Design review of the part built by this model. Coordinates are the model's own, in mm. Face numbers are marked on the shaded views. A direction names the side the tool comes from. Coordinates: 2 decimals unless noted, no trailing zeros. Write each loop counter-clockwise with the first axis right and the second up, starting at its lowest first coordinate (ties: lowest second). Pieces come first, ordered by that corner, then holes. Notation, with made-up numbers: M 69.5,66.25 L 116.5,66.25 A10 cw 116.5,79.25 Z; hole C 30,53 d6. An arc over 180 degrees is marked long. Return JSON: item names as keys, results as strings. Group by question number.
```python
from build123d import *

# Parameters (mm, degrees)
F1_DEPTH = 2
F3_DEPTH = 13
F4_W     = 5
F4_H     = 16
F5_DEPTH = 25
F6_R     = 4


with BuildPart() as f1:
    # F0 (on Top) → F1 (new body)
    with BuildSketch(Plane.XY):
        with BuildLine():
            ThreePointArc((0, -12), (-12, 5e-09), (9.9e-09, 12))
            Line((9.9e-09, 12), (-17, 12))
            Line((-17, 12), (-17, -12))
            Line((-17, -12), (0, -12))
        make_face()
        with BuildLine():
            ThreePointArc((0, -12), (8.4852813742, -8.4852813742), (12, 0))
            ThreePointArc((12, 0), (8.4852813777, 8.4852813707), (9.9e-09, 12))
            ThreePointArc((9.9e-09, 12), (-12, 5e-09), (0, -12))
        make_face()
    extrude(amount=F1_DEPTH)

    # F2 (on face) → F3 (join)
    with BuildSketch(Plane.XY.offset(2)):
        with BuildLine():
            Line((-13, 8), (0, 8))
            Line((0, 8), (8.94427191, 8))
            ThreePointArc((8.94427191, 8), (4.8989794901, 10.9544511481), (9.9e-09, 12))
            Line((9.9e-09, 12), (-17, 12))
            Line((-17, 12), (-17, -12))
            Line((-17, -12), (0, -12))
            ThreePointArc((0, -12), (4.8989794856, -10.9544511501), (8.94427191, -8))
            Line((8.94427191, -8), (0, -8))
            Line((0, -8), (-13, -8))
            Line((-13, -8), (-13, 8))
        make_face()
        with BuildLine():
            ThreePointArc((0, 8), (5.6568542495, 5.6568542495), (8, 0))
            ThreePointArc((8, 0), (5.6568542495, -5.6568542495), (0, -8))
            Line((0, -8), (8.94427191, -8))
            ThreePointArc((8.94427191, -8), (12, 0), (8.94427191, 8))
            Line((8.94427191, 8), (0, 8))
        make_face()
    extrude(amount=F3_DEPTH)

    # F4 (on face) → F5 (cut)
    with BuildSketch(Plane.XY.offset(2)):
        with Locations((-10.5, 0)):
            Rectangle(F4_W, F4_H)
    extrude(amount=-F5_DEPTH, mode=Mode.SUBTRACT)

    # F6
    f6_edges = [f1.edges().sort_by_distance(p)[0] for p in [
        (-17, 12, 7.5),
        (-17, -12, 7.5),
    ]]
    fillet(f6_edges, radius=F6_R)


solid = f1.part
```
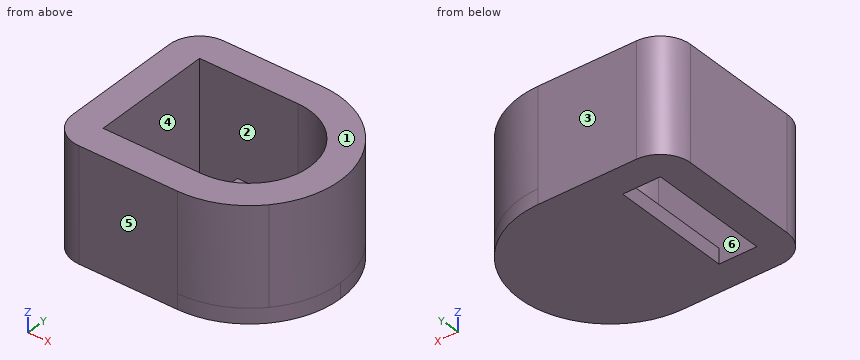
Item 1: For pin 1 (4 mm diameter, centred on y = 3.5, z = 4, fed in from +X); pin 2 (5 mm diameter, centred on x = 7, z = 10, fed in from -Y); pin 3 (8 mm diameter, centred on x = 6.5, z = 6.5, fed in from -Y), all flat-tipped, find the tip position at first contact; note any pin that passes through.
Item 2: Add section A-A (x = -9.5). Write out the cut boundary in (y, z), plus the area to 3 significant figures.
Item 3: Add section D-D (x = -1). Write out the cut boundary in (y, z).
Item 4: Add section C-C (y = 0.5). Write out the cut boundary in (x, z).
Item 5: Add section B-B (z = 7). Write out the cut boundary in (x, y).
Item 6: For line 1 (Y direction, x = -11.75, z = 2.5); line 2 (Y direction, x = 3, z = 14.25); line 3 (Z direction, x = 5.5, y = 2), list the stretches that pass through material, from the lowest coordinate up.
Item 7: The part is to be moulded in two halves that separate along Y. For the marked faces 1, 2 and 3, say which applies: pulls with the +Y half, pulls with the -Y half, needs draft (parallel to the pull), parting line crosses it, or undercut.
Item 8: Machinability: for the marked faces 4, 5 and 6, which of the approach directions +Z, -Z, +X, -X, +Y, -Y give a long, thin tool a straight path to every point of the face, cutting with its end or side? Answer none if there is none.
Geometry check:
{
 "1": {"pin 1": "x = 11.91", "pin 2": "y = -11.12", "pin 3": "y = -11.74"},
 "2": {"outline": "M -12,0 L -8,0 L -8,15 L -12,15 Z; M 8,0 L 12,0 L 12,15 L 8,15 Z", "area": "120 mm^2"},
 "3": {"outline": "M -12,0 L 12,0 L 12,15 L 8,15 L 8,2 L -8,2 L -8,15 L -12,15 Z"},
 "4": {"outline": "M -17,0 L -13,0 L -13,15 L -17,15 Z; M -8,0 L 11.99,0 L 11.99,15 L 7.98,15 L 7.98,2 L -8,2 Z"},
 "5": {"outline": "M -17,-8 A4 ccw -13,-12 L 0,-12 A12 ccw 0,12 L -13,12 A4 ccw -17,8 Z; hole M -13,-8 L 0,-8 A8 ccw 0,8 L -13,8 Z"},
 "6": {"line 1": "-12 to -8, 8 to 12", "line 2": "-11.62 to -7.42, 7.42 to 11.62", "line 3": "0 to 2"},
 "7": {"face 1": "needs draft", "face 2": "undercut", "face 3": "pulls with the +Y half"},
 "8": {"face 4": "+Z, -Z", "face 5": "+Z, -Z, +X, -X, -Y", "face 6": "+Z"}
}
